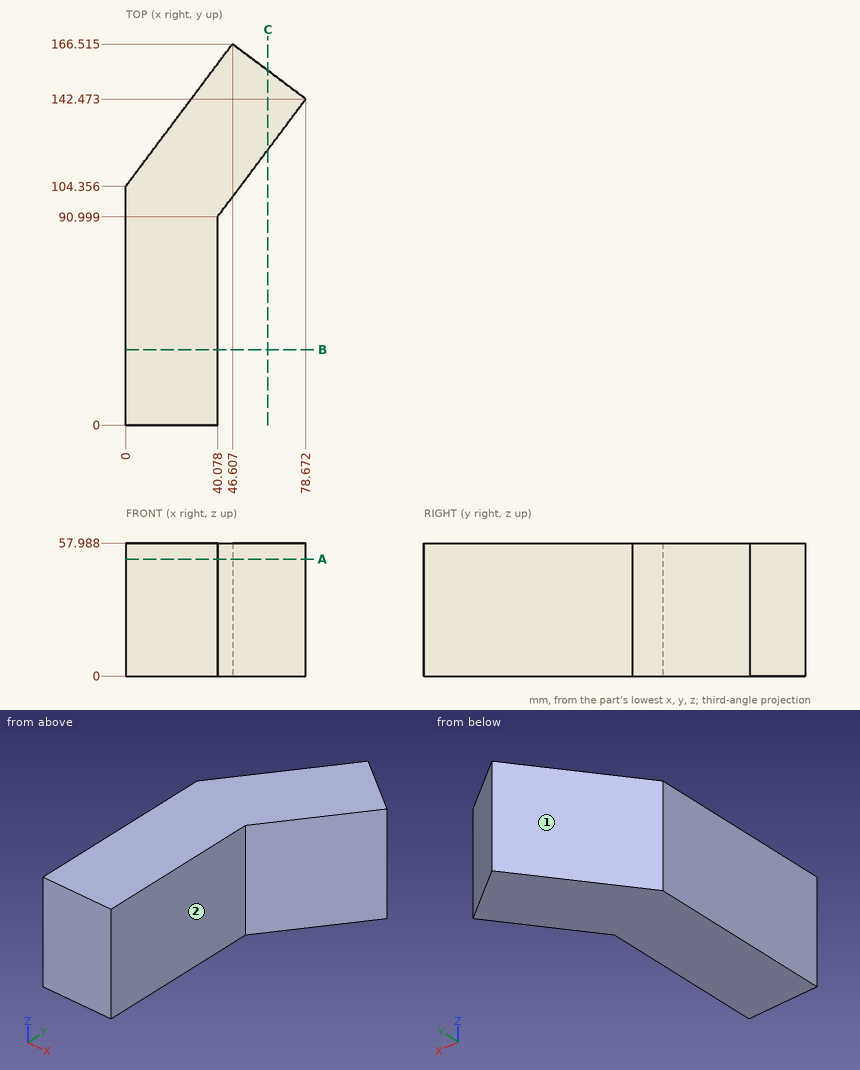
Input: dimensioned drawing with shaded views. Units: mm. Origin: part minimum x, y, z. A direction names the side the tool comes from. Give positions to 0.01 mm unless a question says otherwise; leave off trailing zeros. Order: outer loops, then holes, each group sorted by start corner. A loop starts at its lowest first (then second) coordinate and runs counter-clockwise, first axis right, second up. Notation, with made-up numbers: (10.25, 19.25) -> (62.25, 19.25) arc R20 ccw to (62.25, 43.25) -> close; hole circle Ø9 at (2.5, 81). An arc over 180 degrees is marked (long way). Use a Markdown table: item, result.
1) Section query A-A, the plane z = 51. Return the cut outline in (x, y) (1 decimal), then the cut area to 3 significant figures.
Answer list:
| item | result |
|---|---|
| outline | (0, 0) -> (40.1, 0) -> (40.1, 91) -> (78.7, 142.5) -> (46.6, 166.5) -> (0, 104.4) -> close |
| area | 6,760 mm² |
2) Reachability of the marked faces 1 and 2 from +Z, -Z, +X, -X, +Y, -Y: full face, straight path, thin tool, end or side. Return the list, or none.
Answer list:
| item | result |
|---|---|
| face 1 | +Z, -Z, -X, +Y |
| face 2 | +Z, -Z, +X, -Y |
3) Ray query, line 1 along X through (y, z) = (55.5, 30); line 2 along X through (y, z) = (92.5, 2.5) (1 decimal); line 3 along Y through (x, z) = (52, 50.5). Return the intervals inside material, ascending. Write a range as [from, to].
Answer list:
| item | result |
|---|---|
| line 1 | [0, 40.08] |
| line 2 | [0, 41.2] |
| line 3 | [106.9, 162.47] |
4) Section query B-B, the plane y = 33. Return the cut outline in (x, z), then the cut area to 3 significant figures.
Answer list:
| item | result |
|---|---|
| outline | (0, 0) -> (40.08, 0) -> (40.08, 57.99) -> (0, 57.99) -> close |
| area | 2,320 mm² |
5) Contact query for flat-ended pins moving along their axis: P1, Ø12, axis at x = 12, z = 52, coming from the +Y side; P2, Ø2, axis at x = 31.5, z = 42, coming from the +Y side; P3, Ø2, axis at x = 47, z = 26, coming from the +Y side (1 decimal). Output: stop coordinate, or through.
Answer list:
| item | result |
|---|---|
| P1 | y = 128.36 |
| P2 | y = 147.7 |
| P3 | y = 166.5 |
6) Section query C-C, the plane x = 62. Return the cut outline in (y, z), then the cut area to 3 significant figures.
Answer list:
| item | result |
|---|---|
| outline | (120.24, 0) -> (154.97, 0) -> (154.97, 57.99) -> (120.24, 57.99) -> close |
| area | 2,010 mm² |
